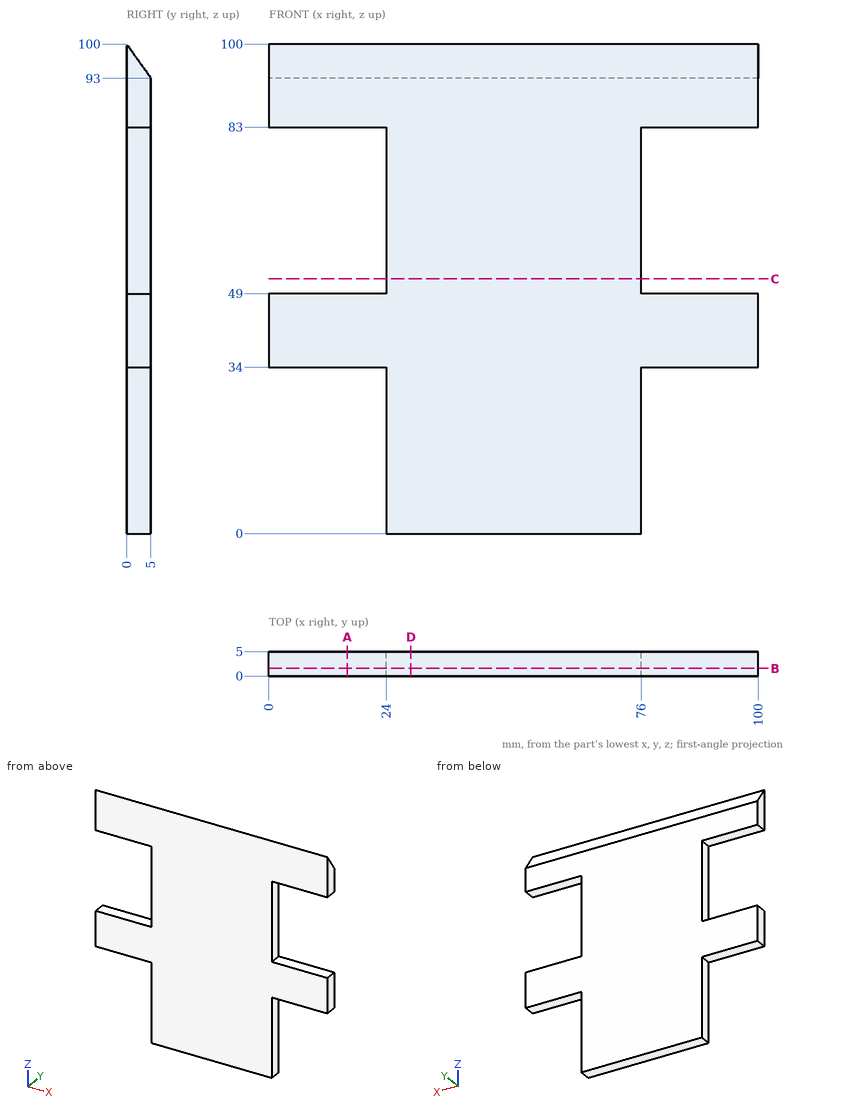
For this review, use the dimensioned drawing (mm, ordinates from the lowest corner) and the shaded views. Coordinates: 2 decimals unless noted, no trailing zeros. Loops run counter-clockwise (first coordinate to the right, second up) from the corner with the lowest first, then second, coordinate; pieces in that order, holes last.
1. For line 1 (X direction, y = 4.1, z = 58.5); line 2 (Z direction, x = 18, y = 2.1); line 3 (Z direction, x = 84, y = 4.45), list the stretches that pass through material, from the lowest coordinate up.
2. Add section D-D, the plane x = 29. Give the boundary of the cut face in (y, z), then the cut area to 4 significant figures.
3. Insertion check: P1, Ø1.5, axis at x = 24.5, y = 3.5, coming from the +Z side; P2, Ø4, axis at x = 29, z = 34.5, coming from the -Y side; P3, Ø1.5, axis at x = 86, y = 2, coming from the -Z side; P4, Ø2.5, axis at y = 3, z = 60, coming from the +X side. Each pin has a flat end and moves straight along its axis. Give the tip position at first contact, or say it passes through.
4. Add section A-A, the plane x = 16. Give the boundary of the cut face in (y, z), then the cut area to 4 significant figures.
5. Add section B-B, the plane y = 1.55. Give the boundary of the cut face in (x, z).
6. Add section C-C, the plane z = 52. Give the boundary of the cut face in (x, y).
Result:
1. line 1: x = 24 to 76
1. line 2: z = 34 to 49, 83 to 97.06
1. line 3: z = 34 to 49, 83 to 93.77
2. outline: (0, 0) - (5, 0) - (5, 93) - (0, 100) - close
2. area: 482.5 mm2
3. P1: stops at z = 96.15
3. P2: stops at y = 0
3. P3: stops at z = 34
3. P4: stops at x = 76
4. outline: (0, 34) - (5, 34) - (5, 49) - (0, 49) - close; (0, 83) - (5, 83) - (5, 93) - (0, 100) - close
4. area: 142.5 mm2
5. outline: (0, 34) - (24, 34) - (24, 0) - (76, 0) - (76, 34) - (100, 34) - (100, 49) - (76, 49) - (76, 83) - (100, 83) - (100, 97.83) - (0, 97.83) - (0, 83) - (24, 83) - (24, 49) - (0, 49) - close
6. outline: (24, 0) - (76, 0) - (76, 5) - (24, 5) - close
